Autodesk Fusion 360 part; units mm, degrees
sketch "Sketch1" plane through (0, 0, 0) normal (0, 0, 1) x (1, 0, 0)
  circle A0 centre (0, 0) radius 3.2
  circle A1 centre (0, 0) radius 6
  line L0 (-3.0605, -0.9346) -> (-5.6926, -1.8959)
  line L1 (-2.5603, 1.9196) -> (-4.3765, 4.1044)
  line L2 (2.5603, 1.9196) -> (4.7149, 3.7108)
  line L3 (2.9267, -1.2939) -> (5.5727, -2.2237)
  dimension "d1" = 6.4
  dimension "d2" = 12
extrude "Extrude1" add sketch "Sketch1" along normal blind 5 contours A0 A1 L2 L3 | A0 A1 L1 L2 | A0 A1 L0 L3 | A0 A1 L0 L1
extrude "Extrude2" add sketch "Sketch1" against normal blind 76 contours A0 A1 L2 L3 | A0 A1 L0 L1
extrude "Extrude3" add sketch "Sketch1" against normal blind 5 from surface at -76 contours A0 A1 L2 L3 | A0 A1 L1 L2 | A0 A1 L0 L3 | A0 A1 L0 L1
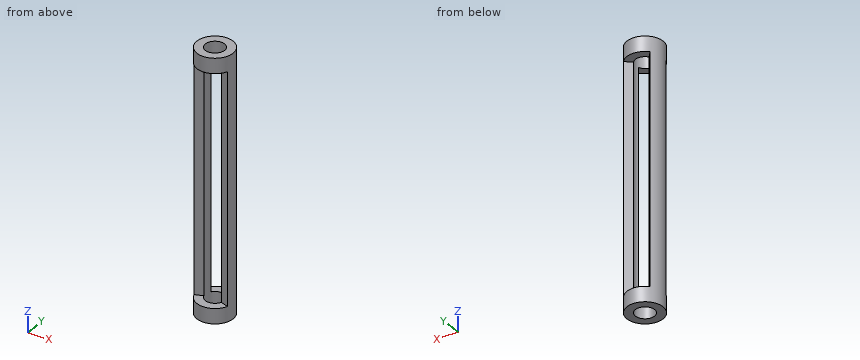
Input: part model. Units: mm. Frame: model coordinates. Give positions to 0.01 mm unless a question says otherwise; leave off trailing zeros. Loops run counter-clockwise (first coordinate to the right, second up) from the corner with the lowest first, then second, coordinate; pieces in that order, holes last.
1) Section query B-B on z = -68. Return the cut outline in (x, y).
A:
outline: (-5.69, -1.9) - (-3.06, -0.93) arc R3.2 cw to (-2.56, 1.92) - (-4.38, 4.1) arc R6 ccw to start; (2.56, 1.92) arc R3.2 cw to (2.93, -1.29) - (5.57, -2.22) arc R6 ccw to (4.71, 3.71) - close
2) Line query: L1, parallel to X at y = 0.25, z = -67; L2, parallel to Z at x = 1.25, y = -4.75; L3, parallel to X at y = -0.75, z = -57. Output: solid intervals per line, ascending.
A:
L1: x = -5.99 to -3.19, 3.19 to 5.99
L2: z = -81 to -76, 0 to 5
L3: x = -5.95 to -3.11, 3.11 to 5.95
3) Section query A-A on x = 0. Return the cut outline in (y, z).
A:
outline: (-6, -81) - (-3.2, -81) - (-3.2, -76) - (-6, -76) - close; (-6, 0) - (-3.2, 0) - (-3.2, 5) - (-6, 5) - close; (3.2, -81) - (6, -81) - (6, -76) - (3.2, -76) - close; (3.2, 0) - (6, 0) - (6, 5) - (3.2, 5) - close
4) Contact query for flat-ended pins moving along their axis: pin 1 (1 mm diameter, centred on y = -1, z = -67, fed in from -X); pin 2 (4 mm diameter, centred on x = 2.5, z = -32.5, fed in from +Y); pin 3 (1.5 mm diameter, centred on x = 2.5, z = -48, fed in from -Y). Output: stop coordinate, or through.
A:
pin 1: stops at x = -5.98
pin 2: stops at y = 3.53
pin 3: stops at y = -1.41
